Source: CAD feature listing. Evaluate the final solid. Frame: model axes, mm. Face numbers are marked on the shaded views. Round coordinates to 2 decimals unless told otherwise and drop trailing zeros. Order: outer loops, then holes, each group sorted by start corner. A loop starts at its lowest first (then second) coordinate and runs counter-clockwise, first axis right, second up. Notation, with made-up numbers: M -25,29.25 L 21,29.25 A15 cw 21,42.25 Z; hole C 68,2 d7. An arc over 180 degrees is marked long. Use one line per item in the form item = value. Start each with the question number.
Q1. Section B-B (y = -1). Return the cut outline in (x, z).
Q2. Section C-C (z = -22.5). Return the cut outline in (x, y).
Q3. Contact query for flat-ended pins moving along their axis: pin 1 (4 mm diameter, centred on x = 12.5, z = -34, fed in from +Y); pin 2 (3 mm diameter, centred on x = 35, z = -30.5, fed in from +Y). Output: stop coordinate, or through.
Q4. Section D-D (x = 22.5). Return the cut outline in (y, z), plus the area to 3 significant figures.
Q5. Pull-direction query (Z, two-part tool) for the marked faces 1 and 2; classes: pulls with the +Z half, pulls with the -Z half, needs draft (parallel to the pull), parting line crosses it, or undercut.
Q6. Material intervals for probe 1 along Z at (x, y) = (11.5, -5); probe 2 along Z at (x, y) = (22, -0.5); probe 3 along Y at (x, z) = (30, -9), sorted ascending.
from build123d import *

# Parameters (mm, degrees)
SKETCH1_W           = 45
SKETCH1_H           = 45
BOSS_EXTRUDE1_DEPTH = 6
SKETCH2_R           = 20
CUT_EXTRUDE1_DEPTH  = 6
CUT_EXTRUDE1_DRAFT  = -60
FILLET2_R           = 2
CUT_EXTRUDE2_DEPTH  = 1000
SKETCH5_W           = 20
SKETCH5_H           = 6
CUT_EXTRUDE3_DEPTH  = 25


with BuildPart() as part:
    # Sketch1 → Boss-Extrude1 (new body)
    with BuildSketch(Plane(origin=(0, 0, 0), x_dir=(1, 0, 0), z_dir=(0, 1, 0))):
        with Locations((22.5, 22.5)):
            Rectangle(SKETCH1_W, SKETCH1_H)
    extrude(amount=-BOSS_EXTRUDE1_DEPTH)


with BuildPart() as cut_extrude1_tool:
    # Sketch2 → Cut-Extrude1 (with draft: the straight prism first)
    with BuildSketch(Plane(origin=(0, 0, 0), x_dir=(1, 0, 0), z_dir=(0, 1, 0))):
        with Locations((22.5, 22.5)):
            Circle(SKETCH2_R)
    extrude(amount=-CUT_EXTRUDE1_DEPTH)
    # Cut-Extrude1: the draft: its side faces are tilted about the plane it starts from
    cut_extrude1_sides = [cut_extrude1_tool.faces().sort_by_distance(p)[0] for p in [
        (2.5, -3, -22.5),
    ]]
    draft(cut_extrude1_sides, Plane(origin=(0, 0, 0), x_dir=(1, 0, 0), z_dir=(0, 1, 0)), CUT_EXTRUDE1_DRAFT)


with BuildPart() as part_1:
    add(part.part)

    # Cut-Extrude1: cut by cut_extrude1_tool
    add(cut_extrude1_tool.part, mode=Mode.SUBTRACT)

    # Fillet2
    fillet2_edges = [part_1.edges().sort_by_distance(p)[0] for p in [
        (22.5, 0, -45),
        (45, 0, -22.5),
        (22.5, 0, 0),
    ]]
    fillet(fillet2_edges, radius=FILLET2_R)

    # Sketch4 → Cut-Extrude2 (cut)
    with BuildSketch(Plane.XY):
        with BuildLine():
            Line((0, 0), (15, 0))
            ThreePointArc((15, 0), (8.107772818, -4.519432044), (0, -6))
            Line((0, -6), (0, 0))
        make_face()
    extrude(amount=-CUT_EXTRUDE2_DEPTH, mode=Mode.SUBTRACT)

    # Sketch5 → Cut-Extrude3 (cut)
    with BuildSketch(Plane(origin=(0, 0, 0), x_dir=(0, 0, -1), z_dir=(1, 0, 0))):
        with Locations((22.5, -3)):
            Rectangle(SKETCH5_W, SKETCH5_H)
    extrude(amount=CUT_EXTRUDE3_DEPTH, mode=Mode.SUBTRACT)


solid = part_1.part
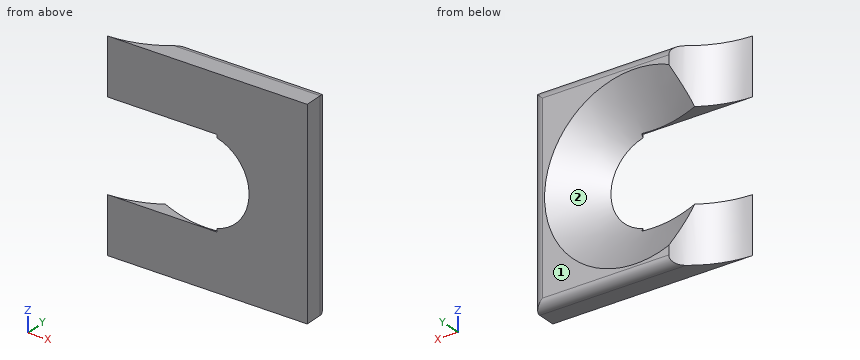
Results list:
q1.outline = M 13.92,-44.73 L 44.73,-44.73 L 44.73,-0.27 L 13.92,-0.27 L 13.92,-6.37 A18.27 cw long 13.92,-38.63 Z
q2.outline = M 32.11,-6 L 45,-6 L 45,-2 A2 ccw 43,0 L 42.5,0 Z
q3.pin_1 = -1.94
q3.pin_2 = -2.11
q4.outline = M -6,-45 L -2,-45 A2 ccw 0,-43 L 0,-42.5 L -5.77,-32.5 L -6,-32.5 Z; M -6,-12.5 L -5.77,-12.5 L 0,-2.5 L 0,-2 A2 ccw -2,0 L -6,0 Z
q4.area = 90.5 mm2
q5.face_1 = needs draft
q5.face_2 = undercut
q6.probe_1 = -45 to -32.5, -12.5 to 0
q6.probe_2 = -44.32 to -41.63, -3.37 to -0.68
q6.probe_3 = -6 to -2.63
